Here's how the part is built. I have some questions about the finished solid (model axes, mm). Round coordinates to 2 decimals unless told otherwise and drop trailing zeros. Order: outer loops, then holes, each group sorted by start corner. A loop starts at its lowest first (then second) coordinate and runs counter-clockwise, first axis right, second up.
```python
from build123d import *

# Parameters (mm, degrees)
F0_W     = 40
F0_H     = 40
F0_R     = 2
F1_DEPTH = 1.5
F2_W     = 40
F2_H     = 40
F3_DEPTH = 25
F4_R     = 4


with BuildPart() as f1:
    # F0 (on Top) → F1 (new body)
    with BuildSketch(Plane.XY):
        Rectangle(F0_W, F0_H)
        with Locations((-16, -16)):
            Circle(F0_R, mode=Mode.SUBTRACT)
        with Locations((16, -16)):
            Circle(F0_R, mode=Mode.SUBTRACT)
        with Locations((-16, 16)):
            Circle(F0_R, mode=Mode.SUBTRACT)
        with Locations((16, 16)):
            Circle(F0_R, mode=Mode.SUBTRACT)
    extrude(amount=F1_DEPTH)

    # F2 (on Top) → F3 (intersect)
    with BuildSketch(Plane.XY):
        Rectangle(F2_W, F2_H)
        with BuildLine():
            Line((-12.540391, -13.601051), (-4.746388, -5.807048))
            ThreePointArc((-4.746388, -5.807048), (-2.870126, -6.929096), (-0.75, -7.462406))
            Line((-0.75, -7.462406), (-0.75, -18.484791))
            ThreePointArc((-0.75, -18.484791), (-7.079643, -17.091771), (-12.540391, -13.601051))
        make_face(mode=Mode.SUBTRACT)
        with BuildLine():
            Line((-18.484791, -0.75), (-7.462406, -0.75))
            ThreePointArc((-7.462406, -0.75), (-6.929096, -2.870126), (-5.807048, -4.746388))
            Line((-5.807048, -4.746388), (-13.601051, -12.540391))
            ThreePointArc((-13.601051, -12.540391), (-17.091771, -7.079643), (-18.484791, -0.75))
        make_face(mode=Mode.SUBTRACT)
        with BuildLine():
            Line((0.75, -18.484791), (0.75, -7.462406))
            ThreePointArc((0.75, -7.462406), (2.870126, -6.929096), (4.746388, -5.807048))
            Line((4.746388, -5.807048), (12.540391, -13.601051))
            ThreePointArc((12.540391, -13.601051), (7.079643, -17.091771), (0.75, -18.484791))
        make_face(mode=Mode.SUBTRACT)
        with BuildLine():
            Line((13.601051, -12.540391), (5.807048, -4.746388))
            ThreePointArc((5.807048, -4.746388), (6.929096, -2.870126), (7.462406, -0.75))
            Line((7.462406, -0.75), (18.484791, -0.75))
            ThreePointArc((18.484791, -0.75), (17.091771, -7.079643), (13.601051, -12.540391))
        make_face(mode=Mode.SUBTRACT)
        with BuildLine():
            ThreePointArc((-18.484791, 0.75), (-17.091771, 7.079643), (-13.601051, 12.540391))
            Line((-13.601051, 12.540391), (-5.807048, 4.746388))
            ThreePointArc((-5.807048, 4.746388), (-6.929096, 2.870126), (-7.462406, 0.75))
            Line((-7.462406, 0.75), (-18.484791, 0.75))
        make_face(mode=Mode.SUBTRACT)
        with BuildLine():
            ThreePointArc((-12.540391, 13.601051), (-7.079643, 17.091771), (-0.75, 18.484791))
            Line((-0.75, 18.484791), (-0.75, 7.462406))
            ThreePointArc((-0.75, 7.462406), (-2.870126, 6.929096), (-4.746388, 5.807048))
            Line((-4.746388, 5.807048), (-12.540391, 13.601051))
        make_face(mode=Mode.SUBTRACT)
        with BuildLine():
            ThreePointArc((13.601051, 12.540391), (17.091771, 7.079643), (18.484791, 0.75))
            Line((18.484791, 0.75), (7.462406, 0.75))
            ThreePointArc((7.462406, 0.75), (6.929096, 2.870126), (5.807048, 4.746388))
            Line((5.807048, 4.746388), (13.601051, 12.540391))
        make_face(mode=Mode.SUBTRACT)
        with BuildLine():
            Line((0.75, 7.462406), (0.75, 18.484791))
            ThreePointArc((0.75, 18.484791), (7.079643, 17.091771), (12.540391, 13.601051))
            Line((12.540391, 13.601051), (4.746388, 5.807048))
            ThreePointArc((4.746388, 5.807048), (2.870126, 6.929096), (0.75, 7.462406))
        make_face(mode=Mode.SUBTRACT)
    extrude(amount=F3_DEPTH, mode=Mode.INTERSECT)

    # F4
    f4_edges = [f1.edges().sort_by_distance(p)[0] for p in [
        (-20, 20, 0.75),
        (20, 20, 0.75),
        (-20, -20, 0.75),
        (20, -20, 0.75),
    ]]
    fillet(f4_edges, radius=F4_R)


solid = f1.part
```
1. If we section it at D-D, the plane z = 1.1: State how many separate pieces and enclosed holes the cut face has, and give its area (3 significant figures).
Evaluation:
separate pieces: 1
enclosed holes: 12
area: 770 mm2
2. If we section it at B-B, the plane x = 9: Write out the boundary of the cut face in (y, z), and give its area (3 significant figures).
Evaluation:
outline: (-20, 0) - (-16.16, 0) - (-16.16, 1.5) - (-20, 1.5) - close; (-10.06, 0) - (-7.94, 0) - (-7.94, 1.5) - (-10.06, 1.5) - close; (-0.75, 0) - (0.75, 0) - (0.75, 1.5) - (-0.75, 1.5) - close; (7.94, 0) - (10.06, 0) - (10.06, 1.5) - (7.94, 1.5) - close; (16.16, 0) - (20, 0) - (20, 1.5) - (16.16, 1.5) - close
area: 20.1 mm2
3. If we section it at C-C, the plane x = -3: Write out the boundary of the cut face in (y, z), and give its area (3 significant figures).
Evaluation:
outline: (-20, 0) - (-18.26, 0) - (-18.26, 1.5) - (-20, 1.5) - close; (-6.87, 0) - (6.87, 0) - (6.87, 1.5) - (-6.87, 1.5) - close; (18.26, 0) - (20, 0) - (20, 1.5) - (18.26, 1.5) - close
area: 25.9 mm2
4. I need wall thicknesses on probe 1 along Y at (x, z) = (-16, 0.7); probe 2 along X at (y, z) = (3.5, 0.15); probe 3 along X at (y, z) = (14.5, 0.6). Which ranges of each line are inside material? Lowest first, please.
Evaluation:
probe 1: y = -20 to -18, -14 to -9.29, -0.75 to 0.75, 9.29 to 14, 18 to 20
probe 2: x = -20 to -18.17, -6.63 to 6.63, 18.17 to 20
probe 3: x = -20 to -17.32, -14.68 to -11.49, -0.75 to 0.75, 11.49 to 14.68, 17.32 to 20
5. If we mould it in two halves opening along Y, with no side actions, what happens to faces 1 (the flat face through (0, -20, 1)), 2 (the cylindrical face through (2.898, 6.917, 0.74))? For each: released by +Y, released by -Y, zero draft, split by the parting line, or undercut.
Evaluation:
face 1: released by -Y
face 2: undercut
6. If we section it at A-A, the plane y = 14.5: Write out the boundary of the cut face in (x, z).
Evaluation:
outline: (-20, 0) - (-17.32, 0) - (-17.32, 1.5) - (-20, 1.5) - close; (-14.68, 0) - (-11.49, 0) - (-11.49, 1.5) - (-14.68, 1.5) - close; (-0.75, 0) - (0.75, 0) - (0.75, 1.5) - (-0.75, 1.5) - close; (11.49, 0) - (14.68, 0) - (14.68, 1.5) - (11.49, 1.5) - close; (17.32, 0) - (20, 0) - (20, 1.5) - (17.32, 1.5) - close
